For this review, take the finished solid that the model builds, in its own axes (mm). A direction names the side the tool comes from. Coordinates: 2 decimals unless noted, no trailing zeros. Order: outer loops, then holes, each group sorted by start corner. A loop starts at its lowest first (then second) coordinate and runs counter-clockwise, first axis right, second up. Notation, with made-up numbers: (11, 44) -> (27, 44) arc R19 cw to (27, 68) -> close; hole circle Ø2 at (73, 17.25). An arc over 180 degrees is marked (long way). Answer as a JSON object with one key per item and string values. Group by question number.
1) Add section B-B, the plane z = -35.5. Write out the cut boundary in (x, y).
2) Add section A-A, the plane y = -157. Write out the cut boundary in (x, z).
3) For pin 1 (1 mm diameter, centred on y = -328.5, z = -54, fed in from -X); pin 2 (1.5 mm diameter, centred on y = 173, z = -31, fed in from +X); pin 3 (21 mm diameter, centred on x = -51, z = -38.5, fed in from -Y), all flat-tipped, find the tip position at first contact; note any pin that passes through.
4) Machinability: for faces 1 (the flat face through (-57, 15, -44)), 2 (the flat face through (-38, -15, 0)), 3 (the flat face through (-38, 15, -44)), which of the approach directions +Z, -Z, +X, -X, +Y, -Y give a long, thin tool a straight path to every point of the face, cutting with its end or side? Answer none if there is none.
5) Wall thickness on L1, parallel to Z at x = -71, y = -915; L2, parallel to X at y = -110, z = -21; L3, parallel to Y at x = -53.5, z = -22.5: over which ranges is each line inside the solid? List them lowest first.
from build123d import *

# Parameters (mm, degrees)
F0_W     = 75
F0_H     = 19
F1_DEPTH = 1104
F2_W     = 19
F2_H     = 2094
F3_DEPTH = 50


with BuildPart() as f1:
    # F0 (on Front) → F1 (new body, symmetric)
    with BuildSketch(Plane.XZ):
        with Locations((-37.5, -9.5)):
            Rectangle(F0_W, F0_H)
    extrude(amount=F1_DEPTH, both=True)

    # F2 (on face) → F3 (join)
    with BuildSketch(Plane(origin=(0, 0, -19), x_dir=(1, 0, 0), z_dir=(0, 0, -1))):
        with Locations((-47.5, 0)):
            Rectangle(F2_W, F2_H)
    extrude(amount=F3_DEPTH)


solid = f1.part
Output values:
{
 "1": {"outline": "(-57, -1047) -> (-38, -1047) -> (-38, 1047) -> (-57, 1047) -> close"},
 "2": {"outline": "(-75, -19) -> (-57, -19) -> (-57, -69) -> (-38, -69) -> (-38, -19) -> (0, -19) -> (0, 0) -> (-75, 0) -> close"},
 "3": {"pin 1": "stops at x = -57", "pin 2": "stops at x = -38", "pin 3": "stops at y = -1047"},
 "4": {"face 1": "-Z, -X, +Y, -Y", "face 2": "+Z, +X, -X, +Y, -Y", "face 3": "-Z, +X, +Y, -Y"},
 "5": {"L1": "z = -19 to 0", "L2": "x = -57 to -38", "L3": "y = -1047 to 1047"}
}
